Read the model definition and answer for the solid it produces. Units are mm, in the model's axes. A direction names the side the tool comes from. Give positions to 0.01 mm unless a question says otherwise; leave off trailing zeros. Order: outer loops, then holes, each group sorted by start corner. A loop starts at its lowest first (then second) coordinate and runs counter-clockwise, first axis right, second up. Notation, with made-up numbers: M 81.5,33.25 L 105.5,33.25 A13 ccw 105.5,37.25 Z; hole C 6.5,-31 d1. An arc over 180 degrees is marked long. Write item = value, one per line. Start each with the question number.
from build123d import *

# Parameters (mm, degrees)
BOSS_EXTRUDE2_DEPTH = 8
FILLET1_R           = 15
FILLET2_R           = 20
FILLET3_R           = 10
FILLET4_R           = 2
FILLET5_R           = 5
SKETCH3_R           = 1.5
CUT_EXTRUDE1_DEPTH  = 78.668634045
FILLET6_R           = 8


# Some blends are built 0.0001 mm under size
with BuildPart() as part:
    # Sketch2 → Boss-Extrude2 (new body)
    with BuildSketch(Plane(origin=(0, 0, 0), x_dir=(0, 0, -1), z_dir=(1, 0, 0))):
        Polygon((0, 0), (9.858322093, 0), (9.858322093, 50), (59.789798831, 47.383202188), (59.789798831, 42.383202188), (15.858322093, 44.685553324), (15.858322093, 20), (21.66602455, 20), (21.66602455, -10), (0, -10), align=None)
    extrude(amount=BOSS_EXTRUDE2_DEPTH)

    # Fillet1
    fillet1_edges = [part.edges().sort_by_distance(p)[0] for p in [
        (4, 44.685553324, -15.858322093),
    ]]
    fillet(fillet1_edges, radius=FILLET1_R)

    # Fillet2
    fillet2_edges = [part.edges().sort_by_distance(p)[0] for p in [
        (4, 50, -9.858322093),
    ]]
    fillet(fillet2_edges, radius=FILLET2_R)

    # Fillet3
    # the kernel refuses this fillet: 10 mm, written as the material it adds along each edge
    with BuildSketch(Plane(origin=(0, 20, -15.858322093), x_dir=(0, 0.9999992265968354, -0.0012437064489906054), z_dir=(1, 0, 0))) as fillet3_piece_1:
        with BuildLine():
            CenterArc((9.089422143, -9.992630476), FILLET3_R, 87.800195831, 67.460307547)
            Line((0.007223077, -5.807697966), (-0.90099683, -5.389204715))
            ThreePointArc((-0.90099683, -5.389204715), (-0.996387688, -2.905092689), (-0.999999227, -0.001243706))
            Line((-0.999999227, -0.001243706), (-0.001243706, 0.999999227))
            ThreePointArc((-0.001243706, 0.999999227), (8.877600872, 1.011041911), (9.511650474, 0.999263048))
            Line((9.511650474, 0.999263048), (9.473266081, 0))
        make_face()
    extrude(amount=8)

    # Fillet4
    fillet4_edges = [part.edges().sort_by_distance(p)[0] for p in [
        (4, 47.383202188, -59.789798831),
        (4, 42.383202188, -59.789798831),
    ]]
    fillet(fillet4_edges, radius=FILLET4_R)

    # Fillet5
    fillet5_edges = [part.edges().sort_by_distance(p)[0] for p in [
        (4, -10, 0),
        (4, 0, 0),
    ]]
    fillet(fillet5_edges, radius=FILLET5_R - 0.0001)  # a hair under: the kernel refuses the full size

    # Sketch3 → Cut-Extrude1 (cut, through all)
    with BuildSketch(Plane(origin=(8, 0, 0), x_dir=(0, 0, -1), z_dir=(1, 0, 0))):
        with Locations((4, -5)):
            Circle(SKETCH3_R)
    extrude(amount=-CUT_EXTRUDE1_DEPTH, mode=Mode.SUBTRACT)

    # Fillet6
    fillet6_edges = [part.edges().sort_by_distance(p)[0] for p in [
        (4, -10, -21.66602455),
    ]]
    fillet(fillet6_edges, radius=FILLET6_R)


solid = part.part
1) Find the intervals of material crossed by probe 1 along Y at (x, z) = (4, -30); probe 2 along Y at (x, z) = (2.5, -4); probe 3 along Z at (x, y) = (4.75, 6), in increasing order. Write a range as [from, to].
2) Find section B-B on z = -4. Determine the outline of the cut face in (x, y).
3) Each of these flat-tipped pins is pushed along its axis until it touches: P1, Ø1, axis at x = 1, y = 0, coming from the -Z side; P2, Ø4, axis at x = 6.5, z = -44, coming from the -Y side; P3, Ø5, axis at y = -5, z = -4, coming from the -X side; P4, Ø4, axis at x = 1.5, z = -35.5, coming from the -Y side. Where does it stop, or does it pass through?
4) Find section C-C on z = -43.5. Determine the outline of the cut face in (x, y), plus the area to 3 significant figures.
5) For faces 1 (the face through (3.94, 23.93, -17.29)), 2 (the face through (3.944, 43.166, -44.847)), 3 (the face through (4, 9, -21.666)), 4 (the face through (4, 0, -7)), determine the directions among +Z, -Z, +X, -X, +Y, -Y from which every point of the face is accessible in a straight line to the end or side of a thin tool.
6) For a pull along Z with two mould halves and no side action, classify faces 5 (the face through (4.06, 40.07, -20.87)), 6 (the face through (0, 20, -21)), 7 (the face through (4.06, -4.55, -5.43)), 8 (the face through (4, 14, -9.858)) as pulls with the +Z half, pulls with the -Z half, needs draft (parallel to the pull), parting line crosses it, or undercut.
7) Find section D-D on y = 24. Determine the outline of the cut face in (x, z).
Numbers:
q1.probe_1 = [43.85, 48.92]
q1.probe_2 = [-9.9, -6.5], [-3.5, -0.1]
q1.probe_3 = [-21.67, -9.86]
q2.outline = M 0,-9.9 L 8,-9.9 L 8,-6.5 L 0,-6.5 Z; M 0,-3.5 L 8,-3.5 L 8,-0.1 L 0,-0.1 Z
q3.P1 = -21.67
q3.P2 = 43.11
q3.P3 = 0
q3.P4 = 43.55
q4.outline = M 0,43.24 L 8,43.24 L 8,48.24 L 0,48.24 Z
q4.area = 40.0 mm2
q5.face_1 = -Z, +X, -X
q5.face_2 = +X, -X, -Y
q5.face_3 = -Z, +X, -X, -Y
q5.face_4 = +Z, +X, -X, +Y
q6.face_5 = undercut
q6.face_6 = needs draft
q6.face_7 = undercut
q6.face_8 = pulls with the +Z half
q7.outline = M 0,-17.25 L 8,-17.25 L 8,-9.86 L 0,-9.86 Z
